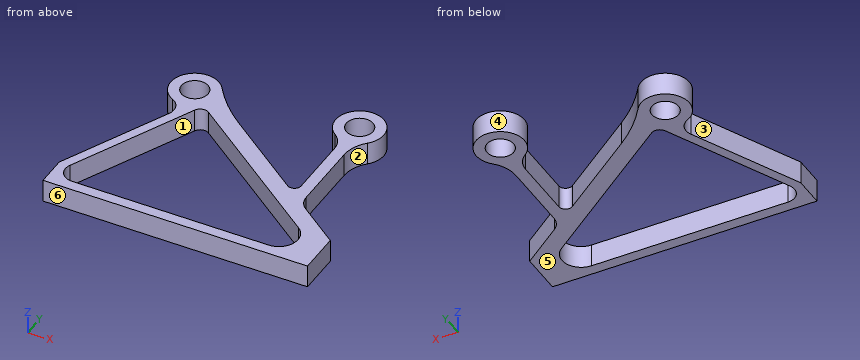
from build123d import *

# Parameters (mm, degrees)
SZKIC2_R                    = 23.25
DODANIE_WYCI_GNI_CIE2_DEPTH = 40


with BuildPart() as part:
    # Szkic2 → Dodanie-wyciągnięcie2 (new body)
    with BuildSketch(Plane.XY):
        with BuildLine():
            Line((356.808690949, 284.085111344), (356.808690949, 175.310171823))
            ThreePointArc((356.808690949, 175.310171823), (350.393476668, 164.898302535), (338.208931835, 165.946569461))
            Line((338.208931835, 165.946569461), (195.757922755, 271.57137534))
            ThreePointArc((195.757922755, 271.57137534), (160.658297297, 302.249297223), (130.912486716, 338.142268))
            ThreePointArc((130.912486716, 338.142268), (64.422832686, 341.168431743), (78.350481289, 276.083469083))
            ThreePointArc((78.350481289, 276.083469083), (91.368118976, 261.595098554), (90.340641348, 242.144749939))
            Line((90.340641348, 242.144749939), (0, 52.788302942))
            Line((0, 52.788302942), (0, 0))
            Line((0, 0), (462, 0))
            Line((462, 0), (461.978142717, 74.173973692))
            Line((461.978142717, 74.173973692), (390.329817514, 127.299890384))
            ThreePointArc((390.329817514, 127.299890384), (380.765620141, 138.664659162), (377.333162938, 153.116305376))
            Line((377.333162938, 153.116305376), (377.333162938, 277.104406009))
            ThreePointArc((377.333162938, 277.104406009), (381.945835927, 300.14062202), (395.072603756, 319.624768565))
            ThreePointArc((395.072603756, 319.624768565), (362.301076624, 391.414618398), (340.803653738, 315.482962688))
            ThreePointArc((340.803653738, 315.482962688), (352.576627129, 301.70602424), (356.808690949, 284.085111344))
        make_face()
        with Locations((96.5, 314)):
            Circle(SZKIC2_R, mode=Mode.SUBTRACT)
        with Locations((365.5, 349.5)):
            Circle(SZKIC2_R, mode=Mode.SUBTRACT)
        with BuildLine():
            Line((142.210331035, 273.398097089), (403.788200613, 79.442912954))
            ThreePointArc((403.788200613, 79.442912954), (415.683061467, 41.906486457), (383.77111031, 18.839228227))
            Line((383.77111031, 18.839228227), (40.223377682, 18.839228227))
            ThreePointArc((40.223377682, 18.839228227), (19.858572573, 30.070249276), (18.491115014, 53.286432871))
            Line((18.491115014, 53.286432871), (120.985954342, 268.118410164))
            ThreePointArc((120.985954342, 268.118410164), (130.352396717, 275.766160753), (142.210331035, 273.398097089))
        make_face(mode=Mode.SUBTRACT)
    extrude(amount=DODANIE_WYCI_GNI_CIE2_DEPTH)


solid = part.part
Here's how the part is built. I have some questions about the finished solid (model axes, mm). Face numbers are marked on the shaded views. A direction names the side the tool comes from. Round coordinates to 2 decimals unless told otherwise and drop trailing zeros. Write each loop counter-clockwise with the first axis right and the second up, starting at its lowest first coordinate (ties: lowest second). Pieces come first, ordered by that corner, then holes. Notation, with made-up numbers: (69, 25) -> (117, 25) arc R6 ccw to (117, 33) -> close; hole circle Ø2 at (48, -33.75). An arc over 180 degrees is marked (long way). One line per item, written item: value.
1) If I drill on line 1 (X direction, y = 300.5, z = 9); line 2 (Y direction, x = 96.5, z = 15); line 3 (Y direction, x = 365.5, z = 20), over which ranges is the centre line in solid material (lowest first)? Write a range as [from, to].
Filled sheet:
line 1: x = [56.69, 77.57], [115.43, 162.38], [353.17, 382.1]
line 2: y = [0, 18.84], [216.8, 290.75], [337.25, 356.04]
line 3: y = [0, 18.84], [107.83, 326.25], [372.75, 391.54]
2) Suppose I cut it at A-A on z = 26. List the corners of the cut face in (x, y) for me.
Filled sheet:
outline: (0, 0) -> (462, 0) -> (461.98, 74.17) -> (390.33, 127.3) arc R32.14 cw to (377.33, 153.12) -> (377.33, 277.1) arc R59.83 cw to (395.07, 319.62) arc R42.04 ccw (long way) to (340.8, 315.48) arc R38.8 cw to (356.81, 284.09) -> (356.81, 175.31) arc R11.66 cw to (338.21, 165.95) -> (195.76, 271.57) arc R290.76 cw to (130.91, 338.14) arc R42.04 ccw (long way) to (78.35, 276.08) arc R25.47 cw to (90.34, 242.14) -> (0, 52.79) -> close; hole (18.49, 53.29) arc R24.08 ccw to (40.22, 18.84) -> (383.77, 18.84) arc R33.61 ccw to (403.79, 79.44) -> (142.21, 273.4) arc R14.17 ccw to (120.99, 268.12) -> close; hole circle Ø46.5 at (96.5, 314); hole circle Ø46.5 at (365.5, 349.5)
3) Suppose I cut it at D-D on y = 25. List the corners of the cut face in (x, z) for me, plus the area to 3 significant figures.
Filled sheet:
outline: (0, 0) -> (24.14, 0) -> (24.14, 40) -> (0, 40) -> close; (403.17, 0) -> (461.99, 0) -> (461.99, 40) -> (403.17, 40) -> close
area: 3,320 mm2
4) Suppose I cut it at C-C on y = 349.5. List the corners of the cut face in (x, z) for me, plus the area to 3 significant figures.
Filled sheet:
outline: (73.99, 0) -> (119.01, 0) -> (119.01, 40) -> (73.99, 40) -> close; (323.46, 0) -> (342.25, 0) -> (342.25, 40) -> (323.46, 40) -> close; (388.75, 0) -> (407.54, 0) -> (407.54, 40) -> (388.75, 40) -> close
area: 3,300 mm2
5) We'd pull the mould along Y, two halves only. Please class the marked faces 4, 5 and 6: released by +Y, released by -Y, zero draft, split by the parting line, or undercut.
Filled sheet:
face 4: undercut
face 5: zero draft
face 6: released by -Y
6) Suppose I cut it at B-B on x = 365.5. List the corners of the cut face in (y, z) for me, plus the area to 3 significant figures.
Filled sheet:
outline: (0, 0) -> (18.84, 0) -> (18.84, 40) -> (0, 40) -> close; (107.83, 0) -> (326.25, 0) -> (326.25, 40) -> (107.83, 40) -> close; (372.75, 0) -> (391.54, 0) -> (391.54, 40) -> (372.75, 40) -> close
area: 10,200 mm2
7) For the marked faces 1, 2 and 3, which set-ups out of +Z, -Z, +X, -X, +Y, -Y let a thin tool reach every point of the face, with its end or its side?
Filled sheet:
face 1: +Z, -Z
face 2: +Z, -Z, +X
face 3: +Z, -Z, -X
8) I'm going to push flat-ended pins straight in: pin 1 Ø3 at (y, z) = (295.5, 18) entering from -X; pin 2 Ø1.5 at (x, z) = (246.5, 24.5) entering from +Y; pin 3 Ø10 at (y, z) = (192.5, 5) entering from -X. Where does each tip first touch, or does it pass through?
Filled sheet:
pin 1: stops at x = 58.05
pin 2: stops at y = 234.5
pin 3: stops at x = 64.27
